Work out the finished part from the listing and answer in its coordinate system (mm). A direction names the side the tool comes from. Coordinates: 2 decimals unless noted, no trailing zeros. Loops run counter-clockwise (first coordinate to the right, second up) from the corner with the lowest first, then second, coordinate; pieces in that order, holes last. Notation, with made-up numbers: (-12.75, 0.25) -> (8.25, 0.25) arc R22 ccw to (8.25, 25.25) -> close; hole circle Ø9 at (66, -5). An arc over 180 degrees is marked (long way). Answer as CSV lines item,"result".
```python
from build123d import *

# Parameters (mm, degrees)
SKETCH1_W                    = 15
SKETCH1_H                    = 57.15
BOSS_EXTRUDE1_DEPTH          = 20
F_6_0_6_DIAMETER_HOLE1_D     = 6
F_6_0_6_DIAMETER_HOLE1_DEPTH = 24
F_6_0_6_DIAMETER_HOLE1_TIP   = 1.802581857
CUT_EXTRUDE1_DEPTH           = 211.546449087


with BuildPart() as part:
    # Sketch1 → Boss-Extrude1 (new body)
    with BuildSketch(Plane.XY):
        with Locations((34.966141976, -180.481947321)):
            Rectangle(SKETCH1_W, SKETCH1_H)
    extrude(amount=BOSS_EXTRUDE1_DEPTH)

    # Ø6.0 (6) Diameter Hole1
    with Locations(Plane(origin=(0, 0, 0), x_dir=(-1, 0, 0), z_dir=(0, 0, -1))):
        with Locations((-34.946141976, -156.986877707), (-34.946141976, -203.976877703)):
            Hole(F_6_0_6_DIAMETER_HOLE1_D / 2, depth=F_6_0_6_DIAMETER_HOLE1_DEPTH)
            with Locations((0, 0, -(F_6_0_6_DIAMETER_HOLE1_DEPTH + F_6_0_6_DIAMETER_HOLE1_TIP / 2))):  # 118° drill point
                Cone(0, F_6_0_6_DIAMETER_HOLE1_D / 2, F_6_0_6_DIAMETER_HOLE1_TIP, mode=Mode.SUBTRACT)

    # Sketch5 → Cut-Extrude1 (cut, through all)
    with BuildSketch(Plane(origin=(42.466141976, 0, 0), x_dir=(0, 0, -1), z_dir=(1, 0, 0))):
        with BuildLine():
            Line((-14.46, -171.629796136), (-14.46, -191.629796136))
            ThreePointArc((-14.46, -191.629796136), (-11.46, -194.629796136), (-8.46, -191.629796136))
            Line((-8.46, -191.629796136), (-8.46, -171.629796136))
            ThreePointArc((-8.46, -171.629796136), (-11.46, -168.629796136), (-14.46, -171.629796136))
        make_face()
    extrude(amount=-CUT_EXTRUDE1_DEPTH, mode=Mode.SUBTRACT)


solid = part.part
```
(1) A cutting plane is placed at B-B, the plane x = 30.75. Write down the section's boundary in (y, z).
Computed values:
outline,"(-209.06, 0) -> (-151.91, 0) -> (-151.91, 20) -> (-209.06, 20) -> close; hole (-191.63, 8.46) -> (-171.63, 8.46) arc R3 ccw to (-171.63, 14.46) -> (-191.63, 14.46) arc R3 ccw to start"
(2) Consider line 1 along Y through (x, z) = (35, 16.75); line 2 along Y through (x, z) = (33.25, 3); line 3 along Y through (x, z) = (37, 9.5). Determine where each line is inside the solid, lowest interval first.
Computed values:
line 1,"-209.06 to -206.98, -200.98 to -159.99, -153.99 to -151.91"
line 2,"-209.06 to -206.45, -201.5 to -159.46, -154.51 to -151.91"
line 3,"-209.06 to -206.16, -201.79 to -193.9, -169.36 to -159.17, -154.8 to -151.91"
(3) A cutting plane is placed at D-D, the plane z = 11.25. Write down the section's boundary in (x, y), and give its area (3 significant figures).
Computed values:
outline,"(27.47, -209.06) -> (42.47, -209.06) -> (42.47, -194.62) -> (27.47, -194.62) -> close; (27.47, -168.64) -> (42.47, -168.64) -> (42.47, -151.91) -> (27.47, -151.91) -> close; hole circle Ø6 at (34.95, -203.98); hole circle Ø6 at (34.95, -156.99)"
area,"411 mm2"
(4) Which of the six approach directions +Z, -Z, +X, -X, +Y, -Y give full straight-line access (tool end or side, diameter ignored) to faces 1 (the face through (34.56, -154.01, 10.14)), 2 (the face through (35.07, -168.63, 11.39))?
Computed values:
face 1,"+Z, -Z"
face 2,"+X, -X"
(5) For a pull along Z with two mould halves and no side action, classify faces 3 (the face through (32.565, -205.802, 10.14)), 4 (the face through (35, -181, 14.46)), 5 (the face through (35, -180, 0)) as pulls with the +Z half, pulls with the -Z half, needs draft (parallel to the pull), parting line crosses it, or undercut.
Computed values:
face 3,"needs draft"
face 4,"undercut"
face 5,"pulls with the -Z half"
(6) A cutting plane is placed at C-C, the plane z = 13.5. Write down the section's boundary in (x, y).
Computed values:
outline,"(27.47, -209.06) -> (42.47, -209.06) -> (42.47, -193.83) -> (27.47, -193.83) -> close; (27.47, -169.43) -> (42.47, -169.43) -> (42.47, -151.91) -> (27.47, -151.91) -> close; hole circle Ø6 at (34.95, -203.98); hole circle Ø6 at (34.95, -156.99)"
(7) A cutting plane is placed at A-A, the plane y = -189.5. Write down the section's boundary in (x, z), and give its area (3 significant figures).
Computed values:
outline,"(27.47, 0) -> (42.47, 0) -> (42.47, 8.46) -> (27.47, 8.46) -> close; (27.47, 14.46) -> (42.47, 14.46) -> (42.47, 20) -> (27.47, 20) -> close"
area,"210 mm2"
(8) A flat-ended cylindrical pin translates along its axis: pin 1 Ø5 at (x, y) = (34.95, -203.98) entering from +Z. Find the tip coordinate at first contact, or state that the pin passes through.
Computed values:
pin 1,"through"
